Input: part model. Units: mm. Frame: model coordinates. Face numbers are marked on the shaded views. A direction names the side the tool comes from. Coordinates: 2 decimals unless noted, no trailing zeros. Loops run counter-clockwise (first coordinate to the right, second up) from the corner with the lowest first, then second, coordinate; pieces in that order, holes last.
Autodesk Inventor part; units mm, degrees
ref_plane "YZ Plane" through (0, 0, 0) normal (1, 0, 0) x (0, 1, 0)
ref_plane "XZ Plane" through (0, 0, 0) normal (0, 1, 0) x (-1, 0, 0)
ref_plane "XY Plane" through (0, 0, 0) normal (0, 0, 1) x (1, 0, 0)
sketch "Sketch1" plane through (0, 0, 0) normal (0, 0, 1) x (1, 0, 0)
  circle A0 centre (0, 0) radius 3.9688
  dimension "d0" = 7.9375
extrude "Extrusion1" add sketch "Sketch1" against normal blind 88.9
sketch "Sketch2" plane through (0, 0, 0) normal (0, 0, 1) x (1, 0, 0)
  circle A0 centre (0, 0) radius 3.9687
  line L0 (-7.3323, 0) -> (-3.6662, 6.35)
  line L1 (-3.6662, 6.35) -> (3.6662, 6.35)
  line L2 (3.6662, 6.35) -> (7.3323, 0)
  line L3 (7.3323, 0) -> (3.6662, -6.35)
  line L4 (3.6662, -6.35) -> (-3.6662, -6.35)
  line L5 (-3.6662, -6.35) -> (-7.3323, 0)
  dimension "d3" = 12.7
extrude "Extrusion2" add sketch "Sketch2" along normal blind 5.1594 contours A0 | L0 L1 L2 L3 L4 L5
thread "Thread1"
chamfer "Chamfer1" distance 0.508 angle 45 1 edges at (-3.9688, 0, -88.9)
fillet "Fillet1" radius 0.508 18 edges at (0, 6.35, 5.1594) (-5.4993, 3.175, 5.1594) (-5.4993, -3.175, 5.1594) (0, -6.35, 5.1594) (5.4993, -3.175, 5.1594) (5.4993, 3.175, 5.1594) (-5.4993, 3.175, 0) (0, 6.35, 0) (5.4993, 3.175, 0) (5.4993, -3.175, 0) (0, -6.35, 0) (-5.4993, -3.175, 0) (7.3323, 0, 2.5797) (3.6662, -6.35, 2.5797) (3.6662, 6.35, 2.5797) (-3.6662, -6.35, 2.5797) (-7.3323, 0, 2.5797) (-3.6662, 6.35, 2.5797)
properties part number "375 bolt x4" material "Steel"
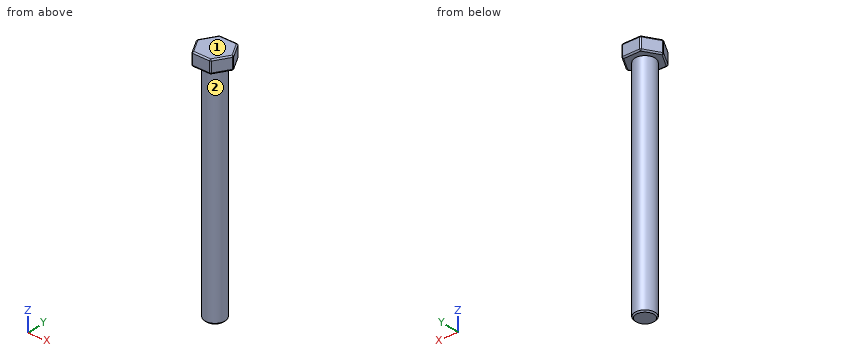
Item 1: Contact query for flat-ended pins moving along their axis: P1, Ø3, axis at x = 5.5, y = -2.5, coming from the +Z side; P2, Ø3, axis at x = 3, z = -44, coming from the +Y side; P3, Ø3, axis at x = 5, z = -30, coming from the +Y side; P4, Ø3, axis at x = -1.5, z = -21, coming from the -Y side. Output: stop coordinate, or through.
Result:
P1: stops at z = 5.16
P2: stops at y = 3.67
P3: stops at y = 1.87
P4: stops at y = -3.97
Item 2: Line query: L1, parallel to Z at x = -3, y = 5; L2, parallel to Y at x = 1.75, z = -75; L3, parallel to X at y = -3, z = -73.5. Output: solid intervals per line, ascending.
Result:
L1: z = 0 to 5.16
L2: y = -3.56 to 3.56
L3: x = -2.6 to 2.6
Item 3: Section query A-A (x = 0). Output: boundary loops of the cut face in (y, z), then the cut area to 3 significant figures.
Result:
outline: (-6.35, 0.51) arc R0.51 ccw to (-5.84, 0) - (-3.97, 0) - (-3.97, -88.39) - (-3.46, -88.9) - (3.46, -88.9) - (3.97, -88.39) - (3.97, 0) - (5.84, 0) arc R0.51 ccw to (6.35, 0.51) - (6.35, 4.65) arc R0.51 ccw to (5.84, 5.16) - (-5.84, 5.16) arc R0.51 ccw to (-6.35, 4.65) - close
area: 771 mm2
Item 4: Reachability of the marked faces 1 and 2 from +Z, -Z, +X, -X, +Y, -Y: full face, straight path, thin tool, end or side. Return the list, or none.
Result:
face 1: +Z, +X, -X, +Y, -Y
face 2: -Z
Item 5: Section query B-B (z = -82.5). Output: boundary loops of the cut face in (x, y).
Result:
outline: circle Ø7.94 at (0, 0)
